```python
from build123d import *

# Parameters (mm, degrees)
SKETCH_1_W           = 16.5
SKETCH_1_H           = 20
EXTRUDE_1_DEPTH      = 7.05
SKETCH_2_W           = 5.3
SKETCH_2_H           = 5.3
EXTRUDE_2_DEPTH      = 9
SKETCH_3_R           = 1.8
CUT_EXTRUDE_1_DEPTH  = 26
SKETCH_4_R           = 2.65
CUT_EXTRUDE_4_DEPTH  = 16
EXTRUDE_3_DEPTH      = 3.65
EXTRUDE_3_DEPTH_BACK = 3.65
EXTRUDE_4_DEPTH      = 1.5
EXTRUDE_4_DEPTH_BACK = 1.5


with BuildPart() as part:
    # 草图1 → 凸台-拉伸1 (new body)
    with BuildSketch(Plane.XY):
        Rectangle(SKETCH_1_W, SKETCH_1_H)
    extrude(amount=EXTRUDE_1_DEPTH)

    # 草图2 → 凸台-拉伸2 (add)
    with BuildSketch(Plane.ZY.offset(8.25)):
        with Locations((3.525, 6.1)):
            Rectangle(SKETCH_2_W, SKETCH_2_H)
        with Locations((3.525, 0)):
            Rectangle(SKETCH_2_W, SKETCH_2_H)
        with Locations((3.525, -6.1)):
            Rectangle(SKETCH_2_W, SKETCH_2_H)
    extrude(amount=EXTRUDE_2_DEPTH)

    # 草图3 → 切除-拉伸1 (cut)
    with BuildSketch(Plane(origin=(8.25, 0, 0), x_dir=(0, 0, -1), z_dir=(1, 0, 0))):
        with Locations((-3.525, 0)):
            Circle(SKETCH_3_R)
        with Locations((-3.525, 6.1)):
            Circle(SKETCH_3_R)
        with Locations((-3.525, -6.1)):
            Circle(SKETCH_3_R)
    extrude(amount=-CUT_EXTRUDE_1_DEPTH, mode=Mode.SUBTRACT)

    # 草图4 → 切除-拉伸4 (cut)
    with BuildSketch(Plane(origin=(8.25, 0, 0), x_dir=(0, 0, -1), z_dir=(1, 0, 0))):
        with Locations((-3.525, 0)):
            Circle(SKETCH_4_R)
        with Locations((-3.525, 6.1)):
            Circle(SKETCH_4_R)
        with Locations((-3.525, -6.1)):
            Circle(SKETCH_4_R)
    extrude(amount=-CUT_EXTRUDE_4_DEPTH, mode=Mode.SUBTRACT)

    # 草图6 → 凸台-拉伸3 (add, two sides: drawn at the far end of the back side and taken through both)
    with BuildSketch(Plane(origin=(0, 0, 0), x_dir=(1, 0, 0), z_dir=(0, 1, 0)).offset(-EXTRUDE_3_DEPTH_BACK)):
        Polygon((-3.205949892, 0.834716435), (5.020511508, 0.834716435), (8.25, 2.067145109), (8.25, 3.607680952), (7.67, 3.607680952), (7.67, 3.027680952), (7.67, 2.466605373), (4.91360258, 1.414716435), (-3.205949892, 1.414716435), (-4.00702853, 1.414716435), (-4.00702853, 0), (-3.205949892, 0), align=None)
    extrude(amount=EXTRUDE_3_DEPTH + EXTRUDE_3_DEPTH_BACK)

    # 草图7 → 凸台-拉伸4 (add, two sides: drawn at the far end of the back side and taken through both)
    with BuildSketch(Plane(origin=(0, 0, 0), x_dir=(1, 0, 0), z_dir=(0, 1, 0)).offset(-EXTRUDE_4_DEPTH_BACK)):
        Polygon((6.29180129, 1.940660904), (-11.289383921, 1.940660904), (-11.289383921, 1.03130852), (-10.541709173, -0.037580686), (-10.541709173, 1.03130852), (-4.00702853, 1.03130852), (-4.00702853, 1.414716435), (4.91360258, 1.414716435), align=None)
    extrude(amount=EXTRUDE_4_DEPTH + EXTRUDE_4_DEPTH_BACK)


solid = part.part
```
Could you check a few things on this model? Use its own coordinates, in mm. A direction names the side the tool comes from. Round coordinates to 2 decimals unless told otherwise and drop trailing zeros. Loops run counter-clockwise (first coordinate to the right, second up) from the corner with the lowest first, then second, coordinate; pieces in that order, holes last. Notation, with made-up numbers: (74, -31) - (113, -31) arc R25 cw to (113, -13) - close; hole circle Ø6 at (63.5, 16.25). An arc over 180 degrees is marked (long way). Use CSV: the item, a comma, the result in double quotes.
Item 1: If we mould it in two halves opening along Y, with no side actions, what happens to faces 1 (the flat face through (0, -10, 3)), 2 (the flat face through (0, 10, 3)), 3 (the flat face through (-13, 3.45, 3)), 4 (the flat face through (-4.007, -0.1, -0.7))? For each: pulls with the +Y half, pulls with the -Y half, needs draft (parallel to the pull), parting line crosses it, or undercut.
Here are the results:
face 1,"pulls with the -Y half"
face 2,"pulls with the +Y half"
face 3,"undercut"
face 4,"needs draft"
Item 2: I need wall thicknesses on L1, parallel to Y at x = -15.25, z = 5.5; L2, parallel to Z at x = -5.25, y = 6; L3, parallel to Y at x = -4.75, z = 5.5. Which ranges of each line are inside material? Lowest first, please. Write a range as [from, to].
Here are the results:
L1,"y = [-8.75, -3.45], [-2.65, 2.65], [3.45, 8.75]"
L2,"z = [0, 0.88], [6.17, 7.05]"
L3,"y = [-10, -7.87], [-4.33, -1.77], [1.77, 4.33], [7.87, 10]"
Item 3: Will these pins go through, and if not, where does the flat tip stop? pin 1 (1.2 mm diameter, centred on y = 0, z = -0.5, fed in from +X); pin 2 (6 mm diameter, centred on x = -14.5, z = 3, fed in from -Y); pin 3 (0.7 mm diameter, centred on y = 0.5, z = -1.5, fed in from -X); pin 4 (4 mm diameter, centred on x = -12.5, y = 6.5, fed in from +Z) (3 decimals).
Here are the results:
pin 1,"stops at x = 8.25"
pin 2,"stops at y = -8.75"
pin 3,"stops at x = -11.29"
pin 4,"stops at z = 6.175"
Item 4: If we section it at B-B on y = 6.1: List the corners of the cut face in (x, z) for me (3 decimals), then the cut area to 3 significant figures.
Here are the results:
outline,"(-17.25, 0.875) - (-8.25, 0.875) - (-8.25, 0) - (8.25, 0) - (8.25, 0.875) - (-7.75, 0.875) - (-7.75, 1.725) - (-17.25, 1.725) - close; (-17.25, 5.325) - (-7.75, 5.325) - (-7.75, 6.175) - (8.25, 6.175) - (8.25, 7.05) - (-8.25, 7.05) - (-8.25, 6.175) - (-17.25, 6.175) - close"
area,"45.0 mm²"
Item 5: If we section it at C-C on x = -11: List the corners of the cut face in (y, z) for me (3 decimals).
Here are the results:
outline,"(-8.75, 0.875) - (-3.45, 0.875) - (-3.45, 6.175) - (-8.75, 6.175) - close; (-2.65, 0.875) - (2.65, 0.875) - (2.65, 6.175) - (-2.65, 6.175) - close; (-1.5, -1.941) - (1.5, -1.941) - (1.5, -0.618) - (-1.5, -0.618) - close; (3.45, 0.875) - (8.75, 0.875) - (8.75, 6.175) - (3.45, 6.175) - close; hole circle Ø3.6 at (-6.1, 3.525); hole circle Ø3.6 at (0, 3.525); hole circle Ø3.6 at (6.1, 3.525)"
Item 6: If we section it at A-A on x = -1.75: List the corners of the cut face in (y, z) for me (3 decimals).
Here are the results:
outline,"(-10, 0) - (10, 0) - (10, 7.05) - (-10, 7.05) - close; (-3.65, -1.415) - (-1.5, -1.415) - (-1.5, -1.941) - (1.5, -1.941) - (1.5, -1.415) - (3.65, -1.415) - (3.65, -0.835) - (-3.65, -0.835) - close; hole circle Ø5.3 at (-6.1, 3.525); hole circle Ø5.3 at (0, 3.525); hole circle Ø5.3 at (6.1, 3.525)"
Item 7: For faces 5 (the cylindrical face through (0.362, -5.983, 6.172)), 6 (the flat face through (-10.92, -0.02, -0.5)), 7 (the flat face through (6.61, -0.05, -1.44)), 8 (the flat face through (-11.289, 0, -1.5)), which set-ups out of +Z, -Z, +X, -X, +Y, -Y let a thin tool reach every point of the face, with its end or its side?
Here are the results:
face 5,"+X"
face 6,"-X, +Y, -Y"
face 7,"+X, +Y, -Y"
face 8,"-Z, -X, +Y, -Y"
